```python
from build123d import *

# Parameters (mm, degrees)
SKETCH1_W           = 42
SKETCH1_H           = 30
BOSS_EXTRUDE1_DEPTH = 15
SKETCH3_R           = 1.5
CUT_EXTRUDE1_DEPTH  = 15
SKETCH4_R           = 5
SKETCH4_R_2         = 4
BOSS_EXTRUDE2_DEPTH = 15
CUT_EXTRUDE2_DEPTH  = 30
CUT_EXTRUDE3_DEPTH  = 30
SKETCH7_R           = 1
CUT_EXTRUDE4_DEPTH  = 30


with BuildPart() as part:
    # Sketch1 → Boss-Extrude1 (new body)
    with BuildSketch(Plane.XY):
        with Locations((21, 15)):
            Rectangle(SKETCH1_W, SKETCH1_H)
    extrude(amount=BOSS_EXTRUDE1_DEPTH)

    # Sketch3 → Cut-Extrude1 (cut)
    with BuildSketch(Plane.XY.offset(15)):
        with Locations((36, 23)):
            Circle(SKETCH3_R)
        with Locations((36, 7)):
            Circle(SKETCH3_R)
    extrude(amount=-CUT_EXTRUDE1_DEPTH, mode=Mode.SUBTRACT)

    # Sketch4 → Boss-Extrude2 (add)
    with BuildSketch(Plane(origin=(42, 0, 0), x_dir=(0, 0, -1), z_dir=(1, 0, 0))):
        with Locations(Location((-7.5, 16, 0), (0, 0, 180))):
            Circle(SKETCH4_R)
        with Locations((-7.5, 16)):
            Circle(SKETCH4_R_2, mode=Mode.SUBTRACT)
    extrude(amount=BOSS_EXTRUDE2_DEPTH)

    # Sketch5 → Cut-Extrude2 (cut)
    with BuildSketch(Plane.XZ):
        with BuildLine():
            Line((24.041336888, 11.530671481), (0, 11.530671481))
            Line((0, 11.530671481), (0, 3.530671481))
            Line((0, 3.530671481), (23.959534392, 3.530671481))
            ThreePointArc((23.959534392, 3.530671481), (31.999738628, 7.448876113), (24.041336888, 11.530671481))
        make_face()
    extrude(amount=-CUT_EXTRUDE2_DEPTH, mode=Mode.SUBTRACT)

    # Sketch6 → Cut-Extrude3 (cut)
    with BuildSketch(Plane.XY.offset(15)):
        with BuildLine():
            ThreePointArc((0, 15), (1.282917549, 22.90569415), (5, 30))
            Line((5, 30), (0, 30))
            Line((0, 30), (0, 15))
        make_face()
        with BuildLine():
            ThreePointArc((5, 0), (1.282917549, 7.09430585), (0, 15))
            Line((0, 15), (0, 0))
            Line((0, 0), (5, 0))
        make_face()
    extrude(amount=-CUT_EXTRUDE3_DEPTH, mode=Mode.SUBTRACT)

    # Sketch7 → Cut-Extrude4 (cut)
    with BuildSketch(Plane.XY.offset(15)):
        with Locations((12, 26)):
            Circle(SKETCH7_R)
        with Locations((12, 4)):
            Circle(SKETCH7_R)
    extrude(amount=-CUT_EXTRUDE4_DEPTH, mode=Mode.SUBTRACT)


solid = part.part
```
The listing builds one solid part. Answer for the finished solid, in the listing's coordinates (mm). A direction names the side the tool comes from. Coordinates: 2 decimals unless noted, no trailing zeros. Write each loop counter-clockwise with the first axis right and the second up, starting at its lowest first coordinate (ties: lowest second). Pieces come first, ordered by that corner, then holes.
Q1. The mould has two halves that part along Z. Classify faces 4 (the cylindrical face through (34.89, 24.01, 7.6)), 5 (the flat face through (12, 15, 11.531)), 6 (the flat face through (21, 15, 15)): released by +Z, released by -Z, zero draft, split by the parting line, or undercut.
Returned:
face 4: zero draft
face 5: undercut
face 6: released by +Z
Q2. Section C-C, the plane y = 4 is taken. Write down the section's boundary in (x, z).
Returned:
outline: (2.55, 0) - (11, 0) - (11, 3.53) - (2.55, 3.53) - close; (2.55, 11.53) - (11, 11.53) - (11, 15) - (2.55, 15) - close; (13, 0) - (42, 0) - (42, 15) - (13, 15) - (13, 11.53) - (24.04, 11.53) arc R5 cw (long way) to (23.96, 3.53) - (13, 3.53) - close
Q3. Given P1, Ø1.5, axis at y = 7, z = 12, coming from the +X side; P2, Ø12, axis at x = 48.5, y = 12, coming from the +Z side; P3, Ø4, axis at y = 10.5, z = 7.5, coming from the -X side, each flat-ended and moving along its own axis, determine where each tip first touches the part or whether it passes through.
Returned:
P1: stops at x = 42
P2: stops at z = 12.5
P3: stops at x = 31.58
Q4. Section A-A, the plane x = 27 is taken. Write down the section's boundary in (y, z), then the cut area to 3 significant figures.
Returned:
outline: (0, 0) - (30, 0) - (30, 2.5) - (0, 2.5) - close; (0, 12.5) - (30, 12.5) - (30, 15) - (0, 15) - close
area: 150 mm2
Q5. Section B-B, the plane x = 36 is taken. Write down the section's boundary in (y, z), then the cut area to 3 significant figures.
Returned:
outline: (0, 0) - (5.5, 0) - (5.5, 15) - (0, 15) - close; (8.5, 0) - (21.5, 0) - (21.5, 15) - (8.5, 15) - close; (24.5, 0) - (30, 0) - (30, 15) - (24.5, 15) - close
area: 360 mm2
Q6. Which of the six approach directions +Z, -Z, +X, -X, +Y, -Y give full straight-line access (tool end or side, diameter ignored) to faces 1 (the cylindrical face through (49.4, 20.88, 6.42)), 2 (the flat face through (27, 30, 2)), 3 (the flat face through (12, 15, 3.531))?
Returned:
face 1: +X
face 2: +Z, -Z, +X, -X, +Y
face 3: -X, +Y, -Y
Q7. Section D-D, the plane z = 5.75 is taken. Write down the section's boundary in (x, y).
Returned:
outline: (31.68, 0) - (42, 0) - (42, 11.32) - (57, 11.32) - (57, 12.4) - (42, 12.4) - (42, 19.6) - (57, 19.6) - (57, 20.68) - (42, 20.68) - (42, 30) - (31.68, 30) - close; hole circle Ø3 at (36, 7); hole circle Ø3 at (36, 23)
Q8. Find the intervals of material crossed by line 1 along Y through (x, z) = (12, 13.45); line 2 along Y through (x, z) = (36, 12.25); line 3 along Z through (x, y) = (13.5, 11), in increasing order.
Returned:
line 1: y = 0 to 3, 5 to 25, 27 to 30
line 2: y = 0 to 5.5, 8.5 to 21.5, 24.5 to 30
line 3: z = 0 to 3.53, 11.53 to 15
